The listing builds one solid part. Answer for the finished solid, in the listing's coordinates (mm). A direction names the side the tool comes from. Coordinates: 2 decimals unless noted, no trailing zeros. Write each loop counter-clockwise with the first axis right and the second up, starting at its lowest first coordinate (ties: lowest second). Pieces come first, ordered by that corner, then holes. Notation, with made-up numbers: M 84,58.5 L 113,58.5 A24 cw 113,73.5 Z; hole C -24,51 d2. An arc over 180 degrees is marked long. Answer as CSV lines item,"result". Start each with the question number.
```python
from build123d import *

# Parameters (mm, degrees)
F1_DEPTH  = 25.4
F2_DEPTH  = 127
F3_W      = 122.7013282478
F3_H      = 129.251409322
F4_DEPTH  = 76.2
F5_DEPTH  = 76.2
F6_DEPTH  = 25.4
F7_R      = 35.9848930873
F8_DEPTH  = 25.4
F9_R      = 44.2111783383
F10_DEPTH = 25.4
F13_R     = 34.5791946556
F12_R     = 32.2271478821
F14_DEPTH = 25.4
F15_R     = 43.299097817
F16_DEPTH = 25.4
F17_R     = 43.1496203252
F18_DEPTH = 25.4
F19_R     = 22.0921612012
F20_DEPTH = 12.7
F21_R     = 45.7423711287
F22_DEPTH = 7.62
F23_DEPTH = 25.4


# Not quite as in the source:
# - a feature names something its author has since deleted; it is built from what else it names


with BuildPart() as f1:
    # F0 (on Front) → F1 (new body)
    with BuildSketch(Plane.XZ):
        Polygon((-46.2158193521, 37.6598188143), (-45.7216948271, 34.3051441014), (-44.4672482626, 31.1548480371), (-42.5201071978, 28.3787638977), (-39.9852425112, 26.1265510978), (-36.9993094144, 24.5196270122), (-33.7232803334, 23.6446213344), (-30.333766844, 23.548705847), (-27.0134984958, 24.2370513787), (-23.9414718147, 25.6725490438), (-21.2833005544, 27.7778107915), (-19.1822874155, 30.4393414161), (-17.7516985602, 33.5136571128), (-17.068657404, 36.8350207265), (-17.1699868723, 40.2243766851), (-18.0502242674, 43.4990039316), (-19.6619157634, 46.4823664636), (-21.9181746546, 49.0136304347), (-24.6973654401, 50.9563347491), (-27.8496612254, 52.2057477143), (-31.2051209287, 52.6945131539), (-34.5828508489, 52.3962815967), (-37.8007566917, 51.3271307829), (-40.6853603202, 49.5446989099), (-43.0811520061, 47.1450773411), (-44.8589739995, 44.2576302965), (-45.9229834566, 41.0380207937), align=None)
    extrude(amount=F1_DEPTH)

    # F2 (add): a face of the model
    f2_faces = [f1.faces().sort_by_distance(p)[0] for p in [
        (-31.618218869, -25.4, 38.0962342024),
    ]]
    extrude(f2_faces, amount=F2_DEPTH)

    # F3 (on Front) → F4 (join)
    with BuildSketch(Plane.XZ):
        with Locations((-1.0198447853, -4.8156213015)):
            Rectangle(F3_W, F3_H)
    extrude(amount=F4_DEPTH)

    # F5 (add): a face of the model
    f5_faces = [f1.faces().sort_by_distance(p)[0] for p in [
        (-1.0198447853, 0, -4.8156213015),
    ]]
    extrude(f5_faces, amount=F5_DEPTH)

    # F6 (add): a face of the model
    f6_faces = [f1.faces().sort_by_distance(p)[0] for p in [
        (-1.0198447853, 0, -69.4413259625),
    ]]
    extrude(f6_faces, amount=F6_DEPTH)

    # F7 (on face) → F8 (join)
    with BuildSketch(Plane.YZ.offset(60.3308193386)):
        with Locations((-53.5847470164, -77.124491334)):
            Circle(F7_R)
    extrude(amount=F8_DEPTH)

    # F9 (on face) → F10 (join)
    with BuildSketch(Plane.YZ.offset(60.3308193386)):
        with Locations((55.2663691342, -70.2658891678)):
            Circle(F9_R)
    extrude(amount=F10_DEPTH)

    # F13 (on face) + F12 (on face) → F14 (join)
    with BuildSketch(Plane(origin=(-62.3705089092, 0, 0), x_dir=(0, -1, 0), z_dir=(-1, 0, 0))):
        with Locations((57.0854917169, -78.4721449018)):
            Circle(F13_R)
    with BuildSketch(Plane(origin=(-62.3705089092, 0, 0), x_dir=(0, -1, 0), z_dir=(-1, 0, 0))):
        with Locations((56.974042207, -73.0006918311)):
            Circle(F12_R)
        with BuildLine():
            Line((76.2, -94.8413259625), (76.2, -47.1365930153))
            ThreePointArc((76.2, -47.1365930153), (33.0171171216, -51.4448387729), (33.2764524277, -94.8413259625))
            Line((33.2764524277, -94.8413259625), (76.2, -94.8413259625))
        make_face()
    extrude(amount=F14_DEPTH)

    # F15 (on face) → F16 (join)
    with BuildSketch(Plane(origin=(-62.3705089092, 0, 0), x_dir=(0, -1, 0), z_dir=(-1, 0, 0))):
        with Locations((-55.8602996171, -70.3753679991)):
            Circle(F15_R)
    extrude(amount=F16_DEPTH)

    # F17 (on face) → F18 (join)
    with BuildSketch(Plane.XY.offset(59.8100833595)):
        Circle(F17_R)
    extrude(amount=F18_DEPTH)

    # F19 (on face) → F20 (join)
    with BuildSketch(Plane.XY.offset(85.2100833595)):
        Circle(F19_R)
    extrude(amount=F20_DEPTH)

    # F21 (on face) → F22 (join)
    with BuildSketch(Plane(origin=(0, 76.2, 0), x_dir=(-1, 0, 0), z_dir=(0, 1, 0))):
        with Locations((0, -36.8642732501)):
            Circle(F21_R)
    extrude(amount=F22_DEPTH)

    # F23 (add): a face of the model
    f23_faces = [f1.faces().sort_by_distance(p)[0] for p in [
        (-31.618218869, -152.4, 38.0962342024),
    ]]
    extrude(f23_faces, amount=F23_DEPTH)


solid = f1.part
```
1) The part is cut by section C-C (y = 0). Determine the outline of the cut face in (x, z), then the cut area to 3 significant figures.
2) The part is cut by section D-D (z = -13.5). Determine the outline of the cut face in (x, y), then the cut area to 3 significant figures.
3) Which of the six approach directions +Z, -Z, +X, -X, +Y, -Y give full straight-line access (tool end or side, diameter ignored) to faces 1 (the face through (60.331, 77, -82)), 2 (the face through (60.331, -61, -95)), 3 (the face through (-16.283, 14.931, 91.471)), 4 (the face through (-74.893, 32.583, -33.865))?
4) Each of these flat-tipped pins is pushed along its axis until it touches: P1, Ø1.5, axis at x = 51.5, z = 42.5, coming from the -Y side; P2, Ø3, axis at x = -19, z = 64.5, coming from the -Y side; P3, Ø2, axis at y = 23.5, z = 6, coming from the -X side. Where does it stop, or does it pass through?
5) The part is cut by section B-B (x = 0). Determine the outline of the cut face in (y, z).
6) Find the intervals of material crossed by line 1 (Z direction, x = -21.5, y = -57.5); line 2 (Y direction, x = 27, z = -28.5); line 3 (X direction, y = 58.5, z = -20.5), in increasing order. Write a range as from..to.
7) The part is cut by section A-A (z = -98). Determine the outline of the cut face in (x, y), then the cut area to 3 significant figures.
8) For a pull along X with two mould halves and no side action, classify faces 5 (the face through (0, 0, 97.91)), 6 (the face through (-2, -76.2, -16)), 7 (the face through (1, 83.82, -36)), 8 (the face through (-5.617, 42.782, 72.332)) as +X half, -X half, draft (parallel to the pull), parting line (faces both ways), or undercut.
Completed:
1,outline,"M -62.37,-94.84 L 60.33,-94.84 L 60.33,59.81 L 43.15,59.81 L 43.15,85.21 L 22.09,85.21 L 22.09,97.91 L -22.09,97.91 L -22.09,85.21 L -43.15,85.21 L -43.15,59.81 L -62.37,59.81 Z"
1,area,"21,700 mm²"
2,outline,"M -62.37,-76.2 L 60.33,-76.2 L 60.33,76.2 L 39.33,76.2 L 39.33,83.82 L -39.33,83.82 L -39.33,76.2 L -62.37,76.2 Z"
2,area,"19,300 mm²"
3,face 1,"-Z, +Y"
3,face 2,"-Z, -Y"
3,face 3,"+Z"
3,face 4,"-X"
4,P1,"y = -76.2"
4,P2,"y = -39.44"
4,P3,"x = -62.37"
5,outline,"M -76.2,-94.84 L 76.2,-94.84 L 76.2,-82.61 L 83.82,-82.61 L 83.82,8.88 L 76.2,8.88 L 76.2,59.81 L 43.15,59.81 L 43.15,85.21 L 22.09,85.21 L 22.09,97.91 L -22.09,97.91 L -22.09,85.21 L -43.15,85.21 L -43.15,59.81 L -76.2,59.81 Z"
6,line 1,"-94.84..59.81"
6,line 2,"-76.2..83.82"
6,line 3,"-62.37..60.33"
7,outline,"M -87.77,-85.62 L -62.37,-85.62 L -62.37,-28.55 L -87.77,-28.55 Z; M -87.77,22.52 L -62.37,22.52 L -62.37,89.2 L -87.77,89.2 Z; M 60.33,-82.9 L 85.73,-82.9 L 85.73,-24.27 L 60.33,-24.27 Z; M 60.33,20.84 L 85.73,20.84 L 85.73,89.7 L 60.33,89.7 Z"
7,area,"6,380 mm²"
8,face 5,"draft"
8,face 6,"undercut"
8,face 7,"undercut"
8,face 8,"parting line"
